Drawing for the job (mm, zero at the part's lowest x, y, z). A direction names the side the tool comes from. Coordinates: 2 decimals unless noted, no trailing zeros. Write each loop counter-clockwise with the first axis right and the second up, starting at its lowest first coordinate (ties: lowest second). Pieces come first, ordered by that corner, then holes. Notation, with made-up numbers: (47, 62) -> (97, 62) arc R24 cw to (97, 88) -> close; hole circle Ø3 at (-31, 48). An arc over 180 degrees is marked (long way). Write each question's results on one line, items separated by ' | '. Start each with the question number.
Q1. Two-plate mould, pull along Y, no slides. Class the marked faces 1, 2 and 3: released by +Y, released by -Y, zero draft, split by the parting line, or undercut.
Q2. Saw through at C-C on y = 9. Give the cut face in (x, z) (3 decimals), and give its area (3 significant figures).
Q3. Drop flat-ended pins along their axis: pin 1 Ø4 at (x, y) = (8, 9.5) entering from +Z; pin 2 Ø3 at (x, y) = (5.5, 8) entering from +Z; pin 3 Ø6.5 at (y, z) = (9, 3.5) entering from -X; pin 4 Ø1.5 at (y, z) = (8, 6.5) entering from -X. Give the stop position or say it passes through.
Q4. Drill centre lines: line 1 (Y direction, x = 7.5, z = 10); line 2 (Z direction, x = 4.25, y = 7.25); line 3 (X direction, y = 13, z = 3). Where is each one in solid material? Low to high.
Q5. Saw through at A-A on x = 6. Give the cut face in (y, z) (3 decimals).
Q6. Tool access for the marked faces 4, 5, 6, 7 and 8: list every direction of +Z, -Z, +X, -X, +Y, -Y with a clear straight run to the whole face (end or side of a thin tool).
Q7. Saw through at B-B on z = 5. Give the cut face in (x, y).
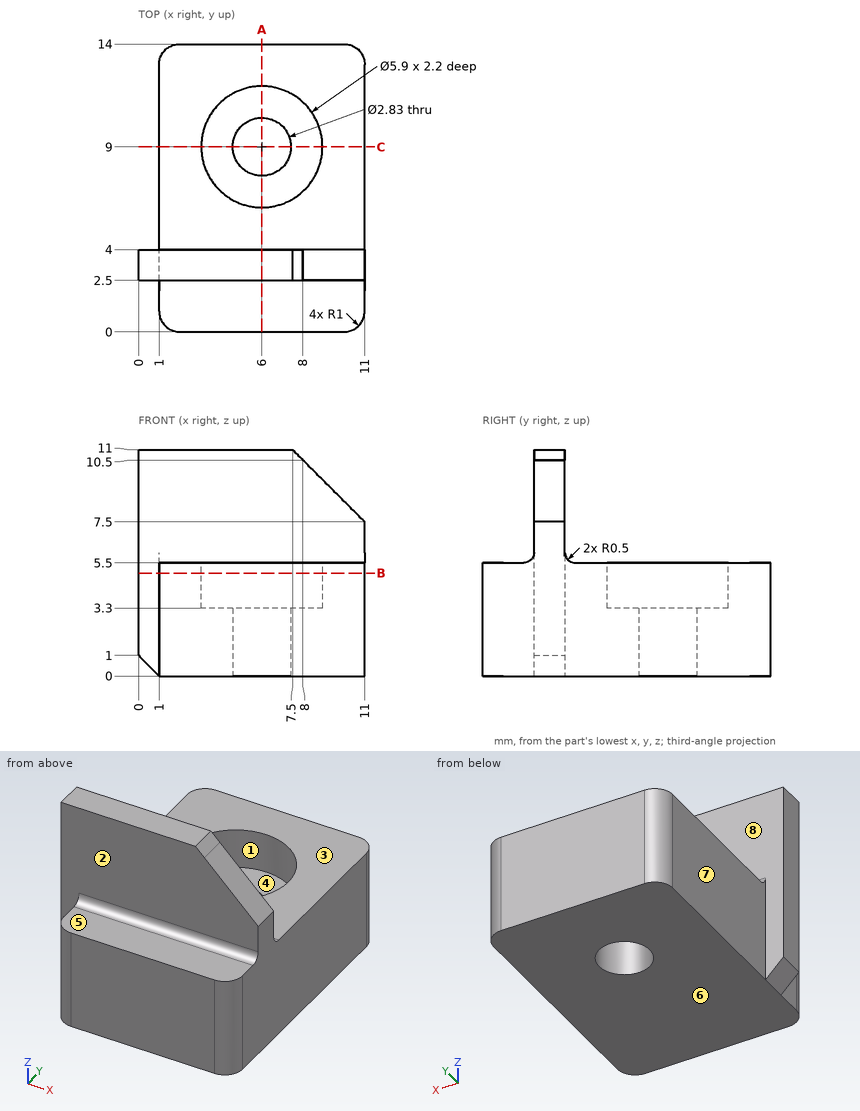
Returned:
1) face 1: undercut | face 2: released by -Y | face 3: zero draft
2) outline: (1, 0) -> (4.585, 0) -> (4.585, 3.3) -> (3.05, 3.3) -> (3.05, 5.5) -> (1, 5.5) -> close; (7.415, 0) -> (11, 0) -> (11, 5.5) -> (8.95, 5.5) -> (8.95, 3.3) -> (7.415, 3.3) -> close | area: 32.7 mm2
3) pin 1: stops at z = 5.5 | pin 2: stops at z = 3.3 | pin 3: stops at x = 1 | pin 4: passes through
4) line 1: y = 2.5 to 4 | line 2: z = 0 to 3.3 | line 3: x = 1 to 11
5) outline: (0, 0) -> (7.585, 0) -> (7.585, 3.3) -> (6.05, 3.3) -> (6.05, 5.5) -> (4.5, 5.5) arc R0.5 cw to (4, 6) -> (4, 11) -> (2.5, 11) -> (2.5, 6) arc R0.5 cw to (2, 5.5) -> (0, 5.5) -> close; (10.415, 0) -> (14, 0) -> (14, 5.5) -> (11.95, 5.5) -> (11.95, 3.3) -> (10.415, 3.3) -> close
6) face 4: +Z | face 5: +Z, +X, -X, -Y | face 6: -Z, +X, -X, +Y, -Y | face 7: +Z, -Z, -X, +Y | face 8: +Z, -X, +Y
7) outline: (0, 2.5) -> (1, 2.5) -> (1, 1) arc R1 ccw to (2, 0) -> (10, 0) arc R1 ccw to (11, 1) -> (11, 13) arc R1 ccw to (10, 14) -> (2, 14) arc R1 ccw to (1, 13) -> (1, 4) -> (0, 4) -> close; hole circle Ø5.9 at (6, 9)
